Read the model definition and answer for the solid it produces. Units are mm, in the model's axes. Face numbers are marked on the shaded views. Coordinates: 2 decimals unless noted, no trailing zeros. Write each loop counter-clockwise with the first axis right and the second up, starting at its lowest first coordinate (ties: lowest second). Pieces come first, ordered by that corner, then holes.
(1) The part is cut by section D-D, the plane x = 13. Determine the outline of the cut face in (y, z).
(2) The part is cut by section C-C, the plane x = 18. Determine the outline of the cut face in (y, z).
(3) Given pin 1 (0.6 mm diameter, centred on y = -3, z = -3, fed in from -X); pin 2 (11.5 mm diameter, centred on x = 0, y = 0, fed in from -Z); pin 3 (1.5 mm diameter, centred on y = 1, z = -1, fed in from +X); pin 4 (1 mm diameter, centred on x = 15, z = -3, fed in from -Y), each flat-ended and moving along its own axis, determine where each tip first touches the part or whether it passes through.
(4) Straight lines are drawn through the part: line 1 along X through (y, z) = (0, -0.6); line 2 along Y through (x, z) = (8, -1.1). For each, find the intervals that lie inside material, in ascending order.
(5) Determine the mould class of the marked faces 1, 2 and 3 for opening direction X: pulls with the +X half, pulls with the -X half, needs draft (parallel to the pull), parting line crosses it, or undercut.
(6) The part is cut by section A-A, the plane x = 0. Determine the outline of the cut face in (y, z).
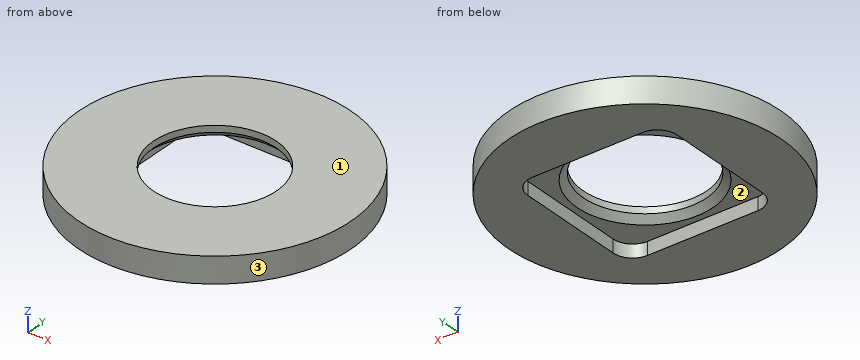
```python
from build123d import *

# Parameters (mm, degrees)
SKETCH001_W  = 11.5
SKETCH001_H  = 4
SKETCH002_W  = 23
SKETCH002_H  = 23
POCKET_DEPTH = 2
FILLET_R     = 3
CHAMFER_SIZE = 1


with BuildPart() as part:
    # Sketch001 → Revolution001 (revolve)
    with BuildSketch(Plane.XZ):
        with Locations((-15.25, -2)):
            Rectangle(SKETCH001_W, SKETCH001_H)
    revolve(axis=Axis((0, 0, 0), (0, 0, 1)))

    # Sketch002 (on Face3 of Revolution001) → Pocket (cut)
    with BuildSketch(Plane(origin=(0, 0, -4), x_dir=(1, 0, 0), z_dir=(0, 0, -1))):
        Rectangle(SKETCH002_W, SKETCH002_H)
    extrude(amount=-POCKET_DEPTH, mode=Mode.SUBTRACT)

    # Fillet
    fillet_edges = [part.edges().sort_by_distance(p)[0] for p in [
        (-11.5, 11.5, -3),
        (11.5, 11.5, -3),
        (11.5, -11.5, -3),
        (-11.5, -11.5, -3),
    ]]
    fillet(fillet_edges, radius=FILLET_R)

    # Chamfer
    chamfer_edges = [part.edges().sort_by_distance(p)[0] for p in [
        (9.5, 0, -2),
    ]]
    chamfer(chamfer_edges, length=CHAMFER_SIZE)


solid = part.part
```
Computed:
1. outline: (-16.49, -4) - (16.49, -4) - (16.49, 0) - (-16.49, 0) - close
2. outline: (-10.82, -4) - (10.82, -4) - (10.82, 0) - (-10.82, 0) - close
3. pin 1: stops at x = -20.83
3. pin 2: passes through
3. pin 3: stops at x = 21
3. pin 4: stops at y = -15.19
4. line 1: x = -21 to -9.5, 9.5 to 21
4. line 2: y = -19.42 to -5.31, 5.31 to 19.42
5. face 1: needs draft
5. face 2: undercut
5. face 3: parting line crosses it
6. outline: (-21, -4) - (-11.5, -4) - (-11.5, -2) - (-10.5, -2) - (-9.5, -1) - (-9.5, 0) - (-21, 0) - close; (9.5, -1) - (10.5, -2) - (11.5, -2) - (11.5, -4) - (21, -4) - (21, 0) - (9.5, 0) - close
